Source: CAD feature listing. Evaluate the final solid. Frame: model axes, mm. A direction names the side the tool comes from. Coordinates: 2 decimals unless noted, no trailing zeros. Order: outer loops, then holes, each group sorted by start corner. A loop starts at its lowest first (then second) coordinate and runs counter-clockwise, first axis right, second up.
Item 1: Mould query, pull axis Y, two halves, no side actions, for faces 4 (the flat face through (-1.465, 29.978, 2.798)), 5 (the flat face through (-1, 58.31, 0)), 6 (the flat face through (-1, -14.906, 0)), 7 (the cylindrical face through (-0.392, -3.176, -0.237)). Classes: released by +Y, released by -Y, zero draft, split by the parting line, or undercut.
Item 2: Reachability of faces 1 (the flat face through (-3.46, 29.98, 2.43)), 2 (the flat face through (-3.8, 29.98, -1.21)), 3 (the flat face through (0.21, 29.98, -3.55)) from +Z, -Z, +X, -X, +Y, -Y: full face, straight path, thin tool, end or side. Return the list, or none.
Item 3: Section A-A on y = 14. Return the cut outline in (x, z).
Item 4: Contact query for flat-ended pins moving along their axis: P1, Ø5, axis at x = -3, y = 38.5, coming from the +Z side; P2, Ø4, axis at y = -5, z = 2.5, coming from the +X side; P3, Ø1.5, axis at y = 20.5, z = -2.5, coming from the +X side. Output: stop coordinate, or through.
Item 5: Ray query, line 1 (Y direction, x = 0.5, z = -1.5); line 2 (Z direction, x = -4, y = 15.5); line 3 (Y direction, x = 0.5, z = -3). Return the intervals inside material, ascending.
from build123d import *

# Parameters (mm, degrees)
BOSS_EXTRUDE1_DEPTH = 60.739130435
SCALE1_SCALE        = 0.92
SKETCH4_R           = 4.953
SKETCH3_R           = 4.953
BOSS_EXTRUDE2_DEPTH = 14.7955
SKETCH5_R           = 2.032
CUT_EXTRUDE1_DEPTH  = 12.957599916


with BuildPart() as part:
    # Sketch1 → Boss-Extrude1 (new body)
    with BuildSketch(Plane(origin=(0, 0, 0), x_dir=(1, 0, 0), z_dir=(0, 1, 0))):
        Polygon((-0.6269783, 2.91618698), (-2.423029524, 4.712238204), (-4.963029524, 2.172238204), (-3.1669783, 0.37618698), (-4.963029524, -1.419864244), (-2.423029524, -3.959864244), (-0.6269783, -2.16381302), (1.169072924, -3.959864244), (3.709072924, -1.419864244), (1.9130217, 0.37618698), (3.709072924, 2.172238204), (1.169072924, 4.712238204), align=None)
    extrude(amount=BOSS_EXTRUDE1_DEPTH)


with BuildPart() as part_1:
    # Scale1: scaled about (-0.6269783, 30.369565217, -0.37618698)
    add(part.part.scale(SCALE1_SCALE).moved(Location((-0.050158264, 2.429565217, -0.030094958))))

    # Sketch4 → section 1 of loft1
    with BuildSketch(Plane(origin=(0, -0.110434783, 0), x_dir=(-1, 0, 0), z_dir=(0, -1, 0)), mode=Mode.PRIVATE) as loft1_s1:
        with Locations((0.6269783, 0.37618698)):
            Circle(SKETCH4_R)
    # loft from a face of the part (loft1)
    loft([part_1.faces().sort_by_distance((-0.6269783, 2.429565217, -0.37618698))[0], loft1_s1.sketch])

    # Sketch3 → Boss-Extrude2 (add)
    with BuildSketch(Plane(origin=(0, -0.110434783, 0), x_dir=(1, 0, 0), z_dir=(0, 1, 0))):
        with Locations((-0.6269783, 0.37618698)):
            Circle(SKETCH3_R)
    extrude(amount=-BOSS_EXTRUDE2_DEPTH)

    # Sketch5 → Cut-Extrude1 (cut, through all)
    with BuildSketch(Plane(origin=(3.376904227, 0, -3.376904227), x_dir=(-0.707106781, 0, -0.707106781), z_dir=(0.707106781, 0, -0.707106781))):
        with Locations((0.709344972, -5.190434783)):
            Circle(SKETCH5_R)
    extrude(amount=-CUT_EXTRUDE1_DEPTH, mode=Mode.SUBTRACT)


solid = part_1.part
Answer list:
1. face 4: zero draft
1. face 5: released by +Y
1. face 6: released by -Y
1. face 7: undercut
2. face 1: +Z, -X, +Y
2. face 2: -X, +Y
2. face 3: -Z, +Y
3. outline: (-4.62, -2.03) - (-2.28, -4.37) - (-0.63, -2.71) - (1.03, -4.37) - (3.36, -2.03) - (1.71, -0.38) - (3.36, 1.28) - (1.03, 3.61) - (-0.63, 1.96) - (-2.28, 3.61) - (-4.62, 1.28) - (-2.96, -0.38) - close
4. P1: stops at z = 3.61
4. P2: stops at x = 4.25
4. P3: stops at x = 3.36
5. line 1: y = -14.91 to -7.22, -3.16 to 58.31
5. line 2: z = -2.64 to -1.41, 0.66 to 1.89
5. line 3: y = -14.91 to -6.93, -3.46 to 58.31
